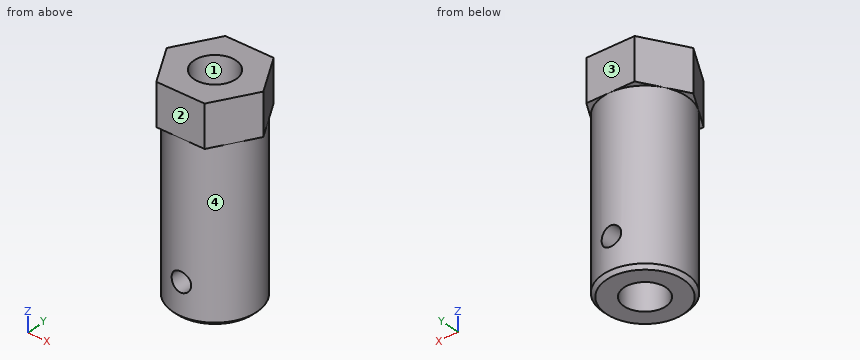
```python
from build123d import *

# Parameters (mm, degrees)
ESQUISSE1_W                  = 24
ESQUISSE1_H                  = 6
BOSS_EXTRU_1_DEPTH           = 6
ENL_V_MAT_EXTRU_1_REACH      = 32
ESQUISSE3_R                  = 3
ESQUISSE4_R                  = 1.400948466
ENL_V_MAT_EXTRU_2_DEPTH      = 7
ENL_V_MAT_EXTRU_2_DEPTH_BACK = 7
CHANFREIN1_SIZE              = 0.5


with BuildPart() as part:
    # Esquisse1 → Révolution1 (revolve)
    with BuildSketch(Plane(origin=(0, 0, 0), x_dir=(0, 0, -1), z_dir=(1, 0, 0))):
        with Locations((-12, 3)):
            Rectangle(ESQUISSE1_W, ESQUISSE1_H)
    revolve(axis=Axis((0, 0, 0), (0, 0, 1)))

    # Esquisse2 → Boss.-Extru.1 (add)
    with BuildSketch(Plane.XY.offset(24)):
        Polygon((6.92820323, 0), (3.464101615, 6), (-3.464101615, 6), (-6.92820323, 0), (-3.464101615, -6), (3.464101615, -6), align=None)
    extrude(amount=BOSS_EXTRU_1_DEPTH)

    # Esquisse3 → Enlèv. mat.-Extru.1 (cut, up to next)
    with BuildSketch(Plane(origin=(0, 0, 0), x_dir=(-1, 0, 0), z_dir=(0, 0, -1)), mode=Mode.PRIVATE) as enl_v_mat_extru_1_sk1:
        Circle(ESQUISSE3_R)
    enl_v_mat_extru_1_tool1 = extrude(enl_v_mat_extru_1_sk1.sketch, amount=-ENL_V_MAT_EXTRU_1_REACH, mode=Mode.PRIVATE) & part.part
    add(enl_v_mat_extru_1_tool1.solids().sort_by_distance((0, 0, 0))[0], mode=Mode.SUBTRACT)

    # Esquisse4 → Enlèv. mat.-Extru.2 (cut, two sides)
    with BuildSketch(Plane(origin=(0, 0, 0), x_dir=(1, 0, 0), z_dir=(0, 1, 0))) as enl_v_mat_extru_2_sk:
        with Locations((0, -5)):
            Circle(ESQUISSE4_R)
    extrude(amount=ENL_V_MAT_EXTRU_2_DEPTH, mode=Mode.SUBTRACT)
    extrude(enl_v_mat_extru_2_sk.sketch, amount=-ENL_V_MAT_EXTRU_2_DEPTH_BACK, mode=Mode.SUBTRACT)

    # Chanfrein1
    chanfrein1_edges = [part.edges().sort_by_distance(p)[0] for p in [
        (0, -6, 0),
    ]]
    chamfer(chanfrein1_edges, length=CHANFREIN1_SIZE)


solid = part.part
```
Geometry check sheet. Reference: the model listing, model coordinates, mm. Face numbers are marked on the shaded views. Give positions to 0.01 mm unless a question says otherwise; leave off trailing zeros. Write each loop counter-clockwise with the first axis right and the second up, starting at its lowest first coordinate (ties: lowest second). Pieces come first, ordered by that corner, then holes.
1) Section check A-A, the plane z = 25. Record the boundary of the cut face in (x, y).
2) Section check B-B, the plane z = 5. Record the boundary of the cut face in (x, y).
3) Section check C-C, the plane z = 17. Record the boundary of the cut face in (x, y), and give its area (3 significant figures).
4) Release check for a two-part mould opening along Y. For the marked faces 1, 2, 3 and 4 record: pulls with the +Y half, pulls with the -Y half, needs draft (parallel to the pull), parting line crosses it, or undercut.
5) Material ranges on L1, parallel to Z at x = 0, y = 4.4; L2, parallel to X at y = -2.5, z = 8.5; L3, parallel to Y at x = 0, z = 14, recorded low to high.
6) Gauge pin test, flat ends, axial feed: pin 1 (0.9 mm diameter, centred on x = 6.5, y = 1.5, fed in from -Z); pin 2 (3.5 mm diameter, centred on x = 4, y = -4, fed in from -Z); pin 3 (1.5 mm diameter, centred on x = -4, z = 5.5, fed in from -Y); pin 4 (4 mm diameter, centred on y = -0.5, z = 21.5, fed in from -X). Record the tip position at first contact, or that the pin passes through.
Computed:
1. outline: (-6.93, 0) - (-3.46, -6) - (3.46, -6) - (6.93, 0) - (3.46, 6) - (-3.46, 6) - close; hole circle Ø6 at (0, 0)
2. outline: (-1.4, -5.83) - (-1.4, -2.65) arc R3 cw to (-1.4, 2.65) - (-1.4, 5.83) arc R6 ccw to start; (1.4, -5.83) arc R6 ccw to (1.4, 5.83) - (1.4, 2.65) arc R3 cw to (1.4, -2.65) - close
3. outline: circle Ø12 at (0, 0); hole circle Ø6 at (0, 0)
3. area: 84.8 mm2
4. face 1: undercut
4. face 2: pulls with the -Y half
4. face 3: pulls with the +Y half
4. face 4: parting line crosses it
5. L1: z = 0 to 3.6, 6.4 to 30
5. L2: x = -5.45 to -1.66, 1.66 to 5.45
5. L3: y = -6 to -3, 3 to 6
6. pin 1: stops at z = 24
6. pin 2: stops at z = 0
6. pin 3: stops at y = -5.04
6. pin 4: stops at x = -6
